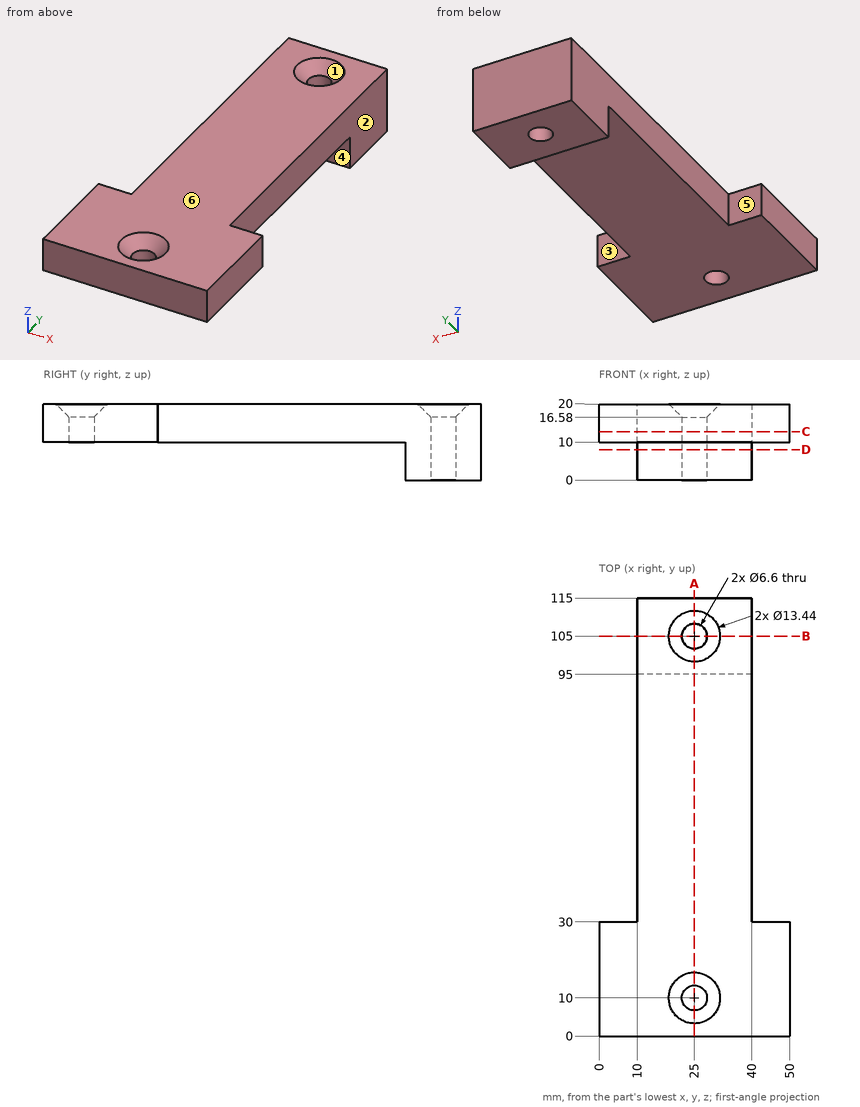
Geometry check sheet. Reference: drawing and pictorial views, mm from the part's lowest x, y, z. A direction names the side the tool comes from. Coordinates: 2 decimals unless noted, no trailing zeros. Write each loop counter-clockwise with the first axis right and the second up, starting at its lowest first coordinate (ties: lowest second). Pieces come first, ordered by that corner, then holes. Notation, with made-up numbers: M 75.5,-10 L 107.5,-10 A25 cw 107.5,14 Z; hole C 74.25,66.25 d7. An arc over 180 degrees is marked long. Write item = value, one per line. Start each with the question number.
1. Sectioned sample at D-D (z = 8). Record the cut outline in (x, y), then the cut area to 3 significant figures.
2. Go/stop test with flat-tipped pins: pin 1 (6 mm diameter, centred on x = 41.5, y = 14.5, fed in from -Z); pin 2 (10 mm diameter, centred on y = 62, z = 10, fed in from +X); pin 3 (11 mm diameter, centred on x = 5.5, z = 16, fed in from +Y); pin 4 (10 mm diameter, centred on y = 92, z = 13, fed in from -X). Record where each tip stops, or that it passes through.
3. Sectioned sample at B-B (y = 105). Record the cut outline in (x, z).
4. Sectioned sample at C-C (z = 12.75). Record the cut outline in (x, y).
5. Thickness scan on probe 1 along Y at (x, z) = (25, 11.75); probe 2 along X at (y, z) = (10, 14); probe 3 along X at (y, z) = (105, 7.5). Record the ranges inside material, lowest first.
6. Mould release check, pull along X, two halves, no side actions. Record for the marked faces 1, 2 and 3: pulls with the +X half, pulls with the -X half, needs draft (parallel to the pull), parting line crosses it, or undercut.
7. Sectioned sample at A-A (x = 25). Record the cut outline in (y, z).
8. Tool access check on the marked faces 4, 5 and 6. Record the directions out of +Z, -Z, +X, -X, +Y, -Y that give a thin tool (end or side, any length) a straight path to the whole face; none if there is none.
The answers:
q1.outline = M 10,95 L 40,95 L 40,115 L 10,115 Z; hole C 25,105 d6.6
q1.area = 566 mm²
q2.pin_1 = 10
q2.pin_2 = 40
q2.pin_3 = 115
q2.pin_4 = 10
q3.outline = M 10,0 L 21.7,0 L 21.7,16.58 L 18.28,20 L 10,20 Z; M 28.3,0 L 40,0 L 40,20 L 31.72,20 L 28.3,16.58 Z
q4.outline = M 0,0 L 50,0 L 50,30 L 40,30 L 40,115 L 10,115 L 10,30 L 0,30 Z; hole C 25,10 d6.6; hole C 25,105 d6.6
q5.probe_1 = 0 to 6.7, 13.3 to 101.7, 108.3 to 115
q5.probe_2 = 0 to 21.7, 28.3 to 50
q5.probe_3 = 10 to 21.7, 28.3 to 40
q6.face_1 = undercut
q6.face_2 = pulls with the +X half
q6.face_3 = needs draft
q7.outline = M 0,10 L 6.7,10 L 6.7,16.58 L 3.28,20 L 0,20 Z; M 13.3,10 L 95,10 L 95,0 L 101.7,0 L 101.7,16.58 L 98.28,20 L 16.72,20 L 13.3,16.58 Z; M 108.3,0 L 115,0 L 115,20 L 111.72,20 L 108.3,16.58 Z
q8.face_4 = -Z, +X, -X, -Y
q8.face_5 = +Z, -Z, -X, +Y
q8.face_6 = +Z, +X, -X, +Y, -Y
